from build123d import *

# Parameters (mm, degrees)
F0_R     = 2.5
F1_DEPTH = 0.5
F3_DEPTH = 11.5
F4_R     = 1.25
F5_DEPTH = 8
F6_SIZE  = 0.25
F7_R     = 1.25
F8_DEPTH = 10


with BuildPart() as f1:
    # F0 (on Top) → F1 (new body)
    with BuildSketch(Plane.XY):
        Circle(F0_R)
    extrude(amount=F1_DEPTH)

    # F2 (on face) → F3 (join)
    with BuildSketch(Plane.XY.offset(0.5)):
        with BuildLine():
            Line((2.5, 0), (2.5, 1.443375673))
            Line((2.5, 1.443375673), (1.2500000021, 2.1650635082))
            ThreePointArc((1.2500000021, 2.1650635082), (2.1650635101, 1.2499999989), (2.5, 0))
        make_face()
        with BuildLine():
            Line((2.5, -1.443375673), (2.5, 0))
            ThreePointArc((2.5, 0), (2.1650635101, -1.2499999989), (1.2500000021, -2.1650635082))
            Line((1.2500000021, -2.1650635082), (2.5, -1.443375673))
        make_face()
        with BuildLine():
            Line((0, -2.8867513459), (1.2500000021, -2.1650635082))
            ThreePointArc((1.2500000021, -2.1650635082), (-1.35e-08, -2.5), (-1.2500000255, -2.1650634947))
            Line((-1.2500000255, -2.1650634947), (0, -2.8867513459))
        make_face()
        with BuildLine():
            Line((-2.5, -1.443375673), (-1.2500000255, -2.1650634947))
            ThreePointArc((-1.2500000255, -2.1650634947), (-2.1650635168, -1.2499999872), (-2.5, 0))
            Line((-2.5, 0), (-2.5, -1.443375673))
        make_face()
        with BuildLine():
            ThreePointArc((-2.5, 0), (-2.1650634924, 1.2500000296), (-1.2499999408, 2.1650635436))
            Line((-1.2499999408, 2.1650635436), (-2.5, 1.443375673))
            Line((-2.5, 1.443375673), (-2.5, 0))
        make_face()
        with BuildLine():
            ThreePointArc((1.2500000021, -2.1650635082), (2.1650635101, -1.2499999989), (2.5, 0))
            ThreePointArc((2.5, 0), (2.1650635101, 1.2499999989), (1.2500000021, 2.1650635082))
            ThreePointArc((1.2500000021, 2.1650635082), (3.54e-08, 2.5), (-1.2499999408, 2.1650635436))
            ThreePointArc((-1.2499999408, 2.1650635436), (-2.1650634924, 1.2500000296), (-2.5, 0))
            ThreePointArc((-2.5, 0), (-2.1650635168, -1.2499999872), (-1.2500000255, -2.1650634947))
            ThreePointArc((-1.2500000255, -2.1650634947), (-1.35e-08, -2.5), (1.2500000021, -2.1650635082))
        make_face()
        with BuildLine():
            ThreePointArc((-1.2499999408, 2.1650635436), (3.54e-08, 2.5), (1.2500000021, 2.1650635082))
            Line((1.2500000021, 2.1650635082), (0, 2.8867513459))
            Line((0, 2.8867513459), (-1.2499999408, 2.1650635436))
        make_face()
    extrude(amount=F3_DEPTH)

    # F4 (on face) → F5 (join)
    with BuildSketch(Plane.XY.offset(12)):
        Circle(F4_R)
    extrude(amount=F5_DEPTH)

    # F6
    f6_edges = [f1.edges().sort_by_distance(p)[0] for p in [
        (-1.25, 0, 20),
    ]]
    chamfer(f6_edges, length=F6_SIZE)

    # F7 (on face) → F8 (cut)
    with BuildSketch(Plane(origin=(0, 0, 0), x_dir=(1, 0, 0), z_dir=(0, 0, -1))):
        Circle(F7_R)
    extrude(amount=-F8_DEPTH, mode=Mode.SUBTRACT)


solid = f1.part
Source: CAD feature listing. Evaluate the final solid. Frame: model axes, mm. A direction names the side the tool comes from. Round coordinates to 2 decimals unless told otherwise and drop trailing zeros. Order: outer loops, then holes, each group sorted by start corner. A loop starts at its lowest first (then second) coordinate and runs counter-clockwise, first axis right, second up. Notation, with made-up numbers: (48, 18) - (60, 18) arc R31 cw to (60, 53) - close; hole circle Ø4 at (45, 17). An arc over 180 degrees is marked (long way). Use a Markdown table: item, result. Add a question column.
1. Section query D-D (y = 1.9). Return the cut outline in (x, z).
2. Section query B-B (x = -2.05). Return the cut outline in (y, z), then the cut area to 3 significant figures.
3. Mould query, pull axis X, two halves, no side actions, for faces 4 (the flat face through (2.5, 0, 6)), 5 (the cylindrical face through (-0.54, -2.44, 0.25)), 6 (the flat face through (0, 0, 20)), 7 (the flat face through (0, 0, 10)). Classes: +X half, -X half, draft (parallel to the pull), parting line (faces both ways), or undercut.
4. Line query: probe 1 along X at (y, z) = (0, 4); probe 2 along Z at (x, y) = (0.6, 1.35); probe 3 along X at (y, z) = (-1, 1.75). Output: solid intervals per line, ascending.
5. Set-up query: faces 1 (the flat face through (-2.295, 1.328, 0.5)), 2 (the cylindrical face through (-0.27, 1.22, 4.93)), 3 (the cylindrical face through (-0.27, -1.22, 15.82)). Return all of +Z, -Z, +X, -X, +Y, -Y with unobstructed straight access to the full face (end or side cutting, diameter ignored); none if empty.
6. Section query A-A (z = 9.5). Return the cut outline in (x, y).
7. Section query C-C (z = 13.75). Return the cut outline in (x, y), then the cut area to 3 significant figures.
8. First-contact query: pin 1 (1 mm diameter, centred on x = 1.5, y = -0.5, fed in from -Z); pin 2 (1.2 mm diameter, centred on x = 0.5, y = 0, fed in from -Z). Flat tips, straight axial feed; report the tip coordinate or a pass-through.
Derived:
| question | item | result |
|---|---|---|
| 1 | outline | (-1.71, 0.5) - (-1.62, 0.5) - (-1.62, 0) - (1.62, 0) - (1.62, 0.5) - (1.71, 0.5) - (1.71, 12) - (-1.71, 12) - close |
| 2 | outline | (-1.7, 0.5) - (-1.43, 0.5) - (-1.43, 0) - (1.43, 0) - (1.43, 0.5) - (1.7, 0.5) - (1.7, 12) - (-1.7, 12) - close |
| 2 | area | 40.6 mm2 |
| 3 | face 4 | +X half |
| 3 | face 5 | parting line |
| 3 | face 6 | draft |
| 3 | face 7 | undercut |
| 4 | probe 1 | -2.5 to -1.25, 1.25 to 2.5 |
| 4 | probe 2 | 0 to 12 |
| 4 | probe 3 | -2.5 to -0.75, 0.75 to 2.5 |
| 5 | face 1 | -Z, -X, +Y |
| 5 | face 2 | -Z |
| 5 | face 3 | +Z |
| 6 | outline | (-2.5, -1.44) - (0, -2.89) - (2.5, -1.44) - (2.5, 1.44) - (0, 2.89) - (-2.5, 1.44) - close; hole circle Ø2.5 at (0, 0) |
| 7 | outline | circle Ø2.5 at (0, 0) |
| 7 | area | 4.91 mm2 |
| 8 | pin 1 | z = 0 |
| 8 | pin 2 | z = 10 |
